The listing builds one solid part. Answer for the finished solid, in the listing's coordinates (mm). A direction names the side the tool comes from. Coordinates: 2 decimals unless noted, no trailing zeros. Order: outer loops, then holes, each group sorted by start corner. A loop starts at its lowest first (then second) coordinate and runs counter-clockwise, first axis right, second up. Notation, with made-up numbers: (-35, -7) - (8, -7) arc R15 cw to (8, 18) - close; hole circle Ø4 at (-31.75, 35.5). An arc over 180 degrees is marked (long way). Use one line per item in the form item = value. Start each with the question number.
Item 1: Section D-D, the plane y = 15.5 is taken. Count the separate pieces of the cut face and the enclosed holes in it, and give its area (3 significant figures).
Item 2: Section B-B, the plane z = 8 is taken. Write down the section's boundary in (x, y).
Item 3: Section C-C, the plane z = -3.25 is taken. Write down the section's boundary in (x, y), and give its area (3 significant figures).
Item 4: Section A-A, the plane x = 0 is taken. Write down the section's boundary in (y, z), and give its area (3 significant figures).
Item 5: A tool of negligible diameter and unlimited length cuts with its end or side. For faces 1 (the flat face through (0, 21.25, -2)), 2 (the flat face through (0, 24.749, -2)), 3 (the cylindrical face through (-17.5, -17, 8)), 4 (the flat face through (-24.749, 0, -2)), from which of +Z, -Z, +X, -X, +Y, -Y can it reach the whole face along a straight path? Write none if from no direction.
Item 6: The mould has two halves that part along X. Classify faces 5 (the flat face through (0, -21.25, -2)), 6 (the flat face through (24.749, 0, -2)), 7 (the flat face through (17, -17, 9)): released by +X, released by -X, zero draft, split by the parting line, or undercut.
Item 7: Consider line 1 along Y through (x, z) = (-15.5, 2); line 2 along X through (y, z) = (20, -2.5); line 3 along Z through (x, y) = (0.5, 6.5). Determine where each line is inside the solid, lowest interval first. Write a range as [from, to].
Item 8: Each of these flat-tipped pins is pushed along its axis until it touches: pin 1 Ø6 at (y, z) = (-15, 4) entering from +X; pin 2 Ø5 at (x, z) = (31.5, 7) entering from -Y; pin 3 Ø1.5 at (x, z) = (10.5, 0) entering from -Y. Where does it stop, or does it pass through?
from build123d import *

# Parameters (mm, degrees)
F0_R     = 42.5
F0_R_2   = 1.5
F0_R_3   = 5
F1_DEPTH = 7
F3_W     = 49.497474
F3_H     = 49.497474
F3_W_2   = 42.5
F3_H_2   = 42.5
F4_DEPTH = 5
F5_R     = 2.5
F5_R_2   = 1.5
F6_DEPTH = 2
F7_R     = 1.5


with BuildPart() as f1:
    # F0 (on Top) → F1 (new body)
    with BuildSketch(Plane.XY):
        Circle(F0_R)
        with Locations((-15.5, -15.5)):
            Circle(F0_R_2, mode=Mode.SUBTRACT)
        with Locations((15.5, -15.5)):
            Circle(F0_R_2, mode=Mode.SUBTRACT)
        with Locations((-15.5, 15.5)):
            Circle(F0_R_2, mode=Mode.SUBTRACT)
        Circle(F0_R_3, mode=Mode.SUBTRACT)
        with Locations((15.5, 15.5)):
            Circle(F0_R_2, mode=Mode.SUBTRACT)
    extrude(amount=F1_DEPTH)

    # F3 (on face) → F4 (join)
    with BuildSketch(Plane(origin=(0, 0, 0), x_dir=(1, 0, 0), z_dir=(0, 0, -1))):
        Rectangle(F3_W, F3_H)
        Rectangle(F3_W_2, F3_H_2, mode=Mode.SUBTRACT)
    extrude(amount=F4_DEPTH)

    # F5 (on offset) → F6 (join)
    with BuildSketch(Plane.XY.offset(7)):
        with Locations((-15.5, 15.5)):
            Circle(F5_R)
        with Locations((-15.5, 15.5)):
            Circle(F5_R_2, mode=Mode.SUBTRACT)
        with Locations((15.5, 15.5)):
            Circle(F5_R)
        with Locations((15.5, 15.5)):
            Circle(F5_R_2, mode=Mode.SUBTRACT)
        with Locations((15.5, -15.5)):
            Circle(F5_R)
        with Locations((15.5, -15.5)):
            Circle(F5_R_2, mode=Mode.SUBTRACT)
        with Locations((-15.5, -15.5)):
            Circle(F5_R)
        with Locations((-15.5, -15.5)):
            Circle(F5_R_2, mode=Mode.SUBTRACT)
    extrude(amount=F6_DEPTH)

    # F7 (on Right) → F8 (revolve, cut)
    with BuildSketch(Plane.YZ):
        with Locations((-39.5, 7.5)):
            Circle(F7_R)
    revolve(axis=Axis((0, 0, 7), (0, 0, 1)), mode=Mode.SUBTRACT)


solid = f1.part
Response:
q1.separate_pieces = 3
q1.enclosed_holes = 0
q1.area = 551 mm2
q2.outline = circle Ø5 at (-15.5, -15.5); circle Ø5 at (-15.5, 15.5); circle Ø5 at (15.5, -15.5); circle Ø5 at (15.5, 15.5); hole circle Ø3 at (-15.5, -15.5); hole circle Ø3 at (-15.5, 15.5); hole circle Ø3 at (15.5, -15.5); hole circle Ø3 at (15.5, 15.5)
q3.outline = (-24.75, -24.75) - (24.75, -24.75) - (24.75, 24.75) - (-24.75, 24.75) - close; hole (-21.25, -21.25) - (21.25, -21.25) - (21.25, 21.25) - (-21.25, 21.25) - close
q3.area = 644 mm2
q4.outline = (-42.5, 0) - (-24.75, 0) - (-24.75, -5) - (-21.25, -5) - (-21.25, 0) - (-5, 0) - (-5, 7) - (-38.09, 7) arc R1.5 cw to (-40.91, 7) - (-42.5, 7) - close; (5, 0) - (21.25, 0) - (21.25, -5) - (24.75, -5) - (24.75, 0) - (42.5, 0) - (42.5, 7) - (40.91, 7) arc R1.5 cw to (38.09, 7) - (5, 7) - close
q4.area = 556 mm2
q5.face_1 = -Z
q5.face_2 = -Z, +X, -X, +Y
q5.face_3 = +Z
q5.face_4 = -Z, -X, +Y, -Y
q6.face_5 = undercut
q6.face_6 = released by +X
q6.face_7 = zero draft
q7.line_1 = [-39.57, -17], [-14, 14], [17, 39.57]
q7.line_2 = [-24.75, -21.25], [21.25, 24.75]
q7.line_3 = [0, 7]
q8.pin_1 = 40.77
q8.pin_2 = -31.07
q8.pin_3 = -41.37
